from build123d import *

# Parameters (mm, degrees)
SKETCH_1_R          = 32.5
EXTRUDE_1_DEPTH     = 15
SKETCH_2_R          = 1.6
CUT_EXTRUDE_1_DEPTH = 27
CUT_EXTRUDE_2_DEPTH = 15
FILLET_1_R          = 5
FILLET_2_R          = 2
CUT_EXTRUDE_START   = 10
SKETCH_4_R          = 24
CUT_EXTRUDE_3_DEPTH = 10
SKETCH_5_R          = 2.5
CUT_EXTRUDE_4_DEPTH = 10


with BuildPart() as part:
    # 草图1 → 凸台-拉伸1 (new body)
    with BuildSketch(Plane(origin=(0, 0, 0), x_dir=(1, 0, 0), z_dir=(0, 1, 0))):
        with Locations(Location((0, 0, 0), (0, 0, 270))):
            Circle(SKETCH_1_R)
    extrude(amount=EXTRUDE_1_DEPTH)

    # 草图2 → 切除-拉伸1 (cut)
    with BuildSketch(Plane(origin=(0, 15, 0), x_dir=(1, 0, 0), z_dir=(0, 1, 0))):
        with Locations(Location((7, 0, 0), (0, 0, 270))):
            Circle(SKETCH_2_R)
        with Locations(Location((0, -7, 0), (0, 0, 270))):
            Circle(SKETCH_2_R)
        with Locations(Location((-7, 0, 0), (0, 0, 270))):
            Circle(SKETCH_2_R)
        with Locations(Location((0, 7, 0), (0, 0, 270))):
            Circle(SKETCH_2_R)
    extrude(amount=-CUT_EXTRUDE_1_DEPTH, mode=Mode.SUBTRACT)

    # 草图3 → 切除-拉伸2 (cut)
    with BuildSketch(Plane(origin=(0, 15, 0), x_dir=(1, 0, 0), z_dir=(0, 1, 0))):
        with BuildLine():
            Line((7, 22.956480566), (7, 7))
            Line((7, 7), (22.956480566, 7))
            ThreePointArc((22.956480566, 7), (16.970562748, 16.970562748), (7, 22.956480566))
        make_face()
        with BuildLine():
            Line((-7, 7), (-22.956480566, 7))
            ThreePointArc((-22.956480566, 7), (-16.970562748, 16.970562748), (-7, 22.956480566))
            Line((-7, 22.956480566), (-7, 7))
        make_face()
        with BuildLine():
            Line((7, -7), (22.956480566, -7))
            ThreePointArc((22.956480566, -7), (16.970562748, -16.970562748), (7, -22.956480566))
            Line((7, -22.956480566), (7, -7))
        make_face()
        with BuildLine():
            Line((-7, -7), (-22.956480566, -7))
            ThreePointArc((-22.956480566, -7), (-16.970562748, -16.970562748), (-7, -22.956480566))
            Line((-7, -22.956480566), (-7, -7))
        make_face()
    extrude(amount=-CUT_EXTRUDE_2_DEPTH, mode=Mode.SUBTRACT)

    # 圆角1
    fillet_1_edges = [part.edges().sort_by_distance(p)[0] for p in [
        (-7, 7.5, -7),
        (7, 7.5, 7),
        (-7, 7.5, 7),
        (7, 7.5, -7),
    ]]
    fillet(fillet_1_edges, radius=FILLET_1_R)

    # 圆角2
    fillet_2_edges = [part.edges().sort_by_distance(p)[0] for p in [
        (-7, 7.5, -22.956480566),
        (-22.956480566, 7.5, -7),
        (7, 7.5, 22.956480566),
        (22.956480566, 7.5, 7),
        (-7, 7.5, 22.956480566),
        (-22.956480566, 7.5, 7),
        (7, 7.5, -22.956480566),
        (22.956480566, 7.5, -7),
    ]]
    fillet(fillet_2_edges, radius=FILLET_2_R)

    # 草图4 → 切除-拉伸3 (cut)
    with BuildSketch(Plane(origin=(0, 0, 0), x_dir=(1, 0, 0), z_dir=(0, 1, 0)).offset(CUT_EXTRUDE_START)):
        with Locations(Location((0, 0, 0), (0, 0, 270))):
            Circle(SKETCH_4_R)
    extrude(amount=-CUT_EXTRUDE_3_DEPTH, mode=Mode.SUBTRACT)

    # 草图5 → 切除-拉伸4 (cut)
    with BuildSketch(Plane(origin=(0, 15, 0), x_dir=(1, 0, 0), z_dir=(0, 1, 0))):
        with Locations(Location((0, 0, 0), (0, 0, 270))):
            Circle(SKETCH_5_R)
    extrude(amount=-CUT_EXTRUDE_4_DEPTH, mode=Mode.SUBTRACT)


solid = part.part
Geometry check sheet. Reference: the model listing, model coordinates, mm. A direction names the side the tool comes from. Give positions to 0.01 mm unless a question says otherwise; leave off trailing zeros. Order: outer loops, then holes, each group sorted by start corner. A loop starts at its lowest first (then second) coordinate and runs counter-clockwise, first axis right, second up. Notation, with made-up numbers: M 32.25,-5 L 37.25,-5 A20 cw 37.25,19 Z; hole C -30.75,37.5 d7. An arc over 180 degrees is marked long. Use a Markdown table: item, result.
Item 1: Tool access check on faces 1 (the cylindrical face through (-9, 12, 8)), 2 (the flat face through (-24, 0, -3)), 3 (the flat face through (-5, 10, 0)). Record the directions out of +Z, -Z, +X, -X, +Y, -Y that give a thin tool (end or side, any length) a straight path to the whole face; none if there is none.
Answers follow:
| item | result |
|---|---|
| face 1 | +Y, -Y |
| face 2 | +Z, -Z, +X, -X, -Y |
| face 3 | -Y |
Item 2: Section check A-A (y = 13.5). State how many separate pieces and enclosed holes the cut face has, and give its area (3 significant figures).
Answers follow:
| item | result |
|---|---|
| separate pieces | 1 |
| enclosed holes | 9 |
| area | 2,620 mm2 |
Item 3: Section check D-D (y = 1.5). Record the cut outline in (x, z).
Answers follow:
| item | result |
|---|---|
| outline | C 0,0 d65; hole C 0,0 d48 |
Item 4: Depth check by flat-ended pin: P1, Ø1, axis at y = 11.5, z = 11.5, coming from the -X side; P2, Ø6, axis at y = 2, z = 6, coming from the +X side; P3, Ø2.5, axis at x = -18, y = 13.5, coming from the -Z side; P4, Ø4, axis at x = 0, z = 7, coming from the +Y side. Enter the tip coordinate at first touch or a pass-through.
Answers follow:
| item | result |
|---|---|
| P1 | stops at x = -30.58 |
| P2 | stops at x = 32.36 |
| P3 | stops at z = -27.85 |
| P4 | stops at y = 15 |
Item 5: Section check B-B (z = 0). Record the cut outline in (x, y), and give its area (3 significant figures).
Answers follow:
| item | result |
|---|---|
| outline | M -32.5,0 L -24,0 L -24,10 L -8.6,10 L -8.6,15 L -32.5,15 Z; M -5.4,10 L -2.5,10 L -2.5,15 L -5.4,15 Z; M 2.5,10 L 5.4,10 L 5.4,15 L 2.5,15 Z; M 8.6,10 L 24,10 L 24,0 L 32.5,0 L 32.5,15 L 8.6,15 Z |
| area | 438 mm2 |
Item 6: Material ranges on line 1 along X through (y, z) = (12.1, 0); line 2 along X through (y, z) = (2.5, 0); line 3 along Y through (x, z) = (15.5, 0), recorded low to high.
Answers follow:
| item | result |
|---|---|
| line 1 | x = -32.5 to -8.6, -5.4 to -2.5, 2.5 to 5.4, 8.6 to 32.5 |
| line 2 | x = -32.5 to -24, 24 to 32.5 |
| line 3 | y = 10 to 15 |
Item 7: Draft check along Z on faces 4 (the flat face through (-7, 15, 7)), 5 (the cylindrical face through (8, 12, 9)), 6 (the cylindrical face through (-8, 12, -9)). Enter one of: +Z half, -Z half, draft (parallel to the pull), parting line (faces both ways), or undercut.
Answers follow:
| item | result |
|---|---|
| face 4 | draft |
| face 5 | undercut |
| face 6 | undercut |
Item 8: Section check C-C (x = 0). Record the cut outline in (y, z).
Answers follow:
| item | result |
|---|---|
| outline | M 0,-32.5 L 15,-32.5 L 15,-8.6 L 10,-8.6 L 10,-24 L 0,-24 Z; M 0,24 L 10,24 L 10,8.6 L 15,8.6 L 15,32.5 L 0,32.5 Z; M 10,-5.4 L 15,-5.4 L 15,-2.5 L 10,-2.5 Z; M 10,2.5 L 15,2.5 L 15,5.4 L 10,5.4 Z |
